Autodesk Fusion 360 part; units mm, degrees
sketch "スケッチ1" plane through (0, 0, 0) normal (0, 0, 1) x (1, 0, 0)
  circle A0 centre (0, 0) radius 83
  dimension "d1" = 166
extrude "押し出し1" add sketch "スケッチ1" along normal blind 46
sketch "スケッチ2" plane through (0, 0, 46) normal (0, 0, 1) x (-1, 0, 0)
  circle A0 centre (0, 0) radius 83
  circle A1 centre (0, 0) radius 27.119
extrude "押し出し2" add sketch "スケッチ2" along normal blind 3.5 contours A1
sketch "スケッチ3" plane through (0, 0, 49.5) normal (0, 0, 1) x (-1, 0, 0)
  circle A0 centre (0, 0) radius 27.119
  circle A1 centre (0, 0) radius 6.5
  dimension "d6" = 13
extrude "押し出し3" add sketch "スケッチ3" along normal blind 52.5 contours A1
sketch "スケッチ4" plane through (0, 0, 0) normal (1, 0, 0) x (0, 1, 0)
  line L0 (6.5, 102) -> (-6.5, 102)
  line L1 (-6.5, 49.5) -> (6.5, 49.5)
  line L2 (6.5, 102) -> (6.5, 99)
  line L3 (6.5, 99) -> (3.5, 99)
  line L4 (3.5, 99) -> (3.5, 55)
  line L5 (3.5, 55) -> (6.5, 55)
  line L6 (6.5, 55) -> (6.5, 99)
  dimension "d9" = 3
  dimension "d10" = 44
  dimension "d11" = 3
extrude "押し出し4" cut sketch "スケッチ4" along normal blind 52.5 and the other way blind 60
sketch "スケッチ5" plane through (0, 0, 0) normal (0, 0, -1) x (1, 0, 0)
  circle A0 centre (0, 0) radius 83
  circle A1 centre (0, 0) radius 59.4788
extrude "押し出し5" add sketch "スケッチ5" along normal blind 9.5 contours A1
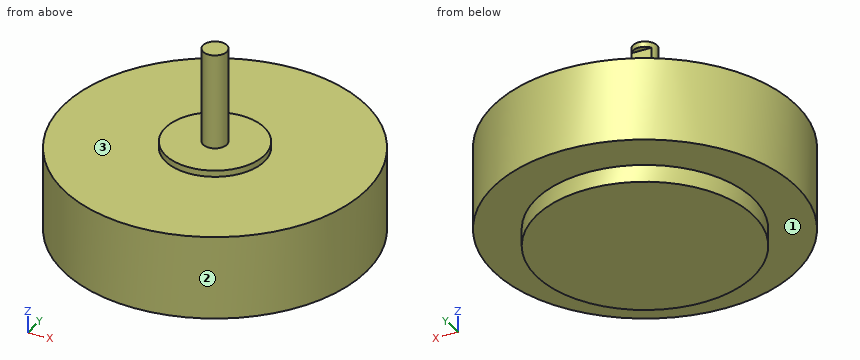
Input: part model. Units: mm. Frame: model coordinates. Face numbers are marked on the shaded views. A direction names the side the tool comes from. Give positions to 0.01 mm unless a question says otherwise; leave off trailing zeros. Order: outer loops, then holes, each group sorted by start corner. A loop starts at its lowest first (then second) coordinate and runs counter-clockwise, first axis right, second up. Notation, with made-up numbers: (33, 83.25) - (92, 83.25) arc R24 ccw to (92, 105.25) - close; hole circle Ø3 at (29.5, 47.25). An arc over 180 degrees is marked (long way). One line per item, written item: value.
1. Cut plane C-C, the plane z = 33. Output: boundary loops of the cut face in (x, y).
Determined:
outline: circle Ø166 at (0, 0)
2. Pin query (flat end, axial travel): pin 1 Ø8 at (x, z) = (-10, 89.5) entering from +Y; pin 2 Ø10 at (y, z) = (23, 45) entering from -X; pin 3 Ø1.5 at (y, z) = (17, 29.5) entering from +X. Return the tip coordinate at first contact, or that it passes through.
Determined:
pin 1: y = 2.5
pin 2: x = -81.02
pin 3: x = 81.39
3. Line query: probe 1 along Z at (x, y) = (41, 13); probe 2 along Z at (x, y) = (-14, 16.5); probe 3 along Y at (x, z) = (-2, 7). Output: solid intervals per line, ascending.
Determined:
probe 1: -9.5 to 46
probe 2: -9.5 to 49.5
probe 3: -82.98 to 82.98
4. Cut plane D-D, the plane y = -57. Output: boundary loops of the cut face in (x, z), and give its area (3 significant figures).
Determined:
outline: (-60.33, 0) - (-16.99, 0) - (-16.99, -9.5) - (16.99, -9.5) - (16.99, 0) - (60.33, 0) - (60.33, 46) - (-60.33, 46) - close
area: 5,870 mm2
5. Cut plane B-B, the plane y = 0. Output: boundary loops of the cut face in (x, z).
Determined:
outline: (-83, 0) - (-59.48, 0) - (-59.48, -9.5) - (59.48, -9.5) - (59.48, 0) - (83, 0) - (83, 46) - (27.12, 46) - (27.12, 49.5) - (6.5, 49.5) - (6.5, 102) - (-6.5, 102) - (-6.5, 49.5) - (-27.12, 49.5) - (-27.12, 46) - (-83, 46) - close
6. Cut plane A-A, the plane x = 0. Output: boundary loops of the cut face in (y, z).
Determined:
outline: (-83, 0) - (-59.48, 0) - (-59.48, -9.5) - (59.48, -9.5) - (59.48, 0) - (83, 0) - (83, 46) - (27.12, 46) - (27.12, 49.5) - (6.5, 49.5) - (6.5, 55) - (3.5, 55) - (3.5, 99) - (6.5, 99) - (6.5, 102) - (-6.5, 102) - (-6.5, 49.5) - (-27.12, 49.5) - (-27.12, 46) - (-83, 46) - close
7. Reachability of the marked faces 1, 2 and 3 from +Z, -Z, +X, -X, +Y, -Y: full face, straight path, thin tool, end or side. Return the list, or none.
Determined:
face 1: -Z
face 2: +Z, -Z
face 3: +Z
